from build123d import *

# Parameters (mm, degrees)
EXTRUDE_1_DEPTH = 2


with BuildPart() as part:
    # 草图2 → 凸台-拉伸1 (new body)
    with BuildSketch(Plane.XY):
        Polygon((-15.2, 6.5), (74.2, 6.5), (74.2, 8.5), (78, 8.5), (78, 6.5), (80.5, 6.5), (80.5, 4), (79, 4), (79, 1.4), (80.5, 1.4), (80.5, -1.6), (83.5, -1.6), (83.5, 1.4), (85, 1.4), (85, 4), (83.5, 4), (83.5, 6.5), (86, 6.5), (86, 8.5), (89.8, 8.5), (89.8, 6.5), (197.54, 6.5), (197.54, 8.5), (201.34, 8.5), (201.34, 6.5), (203.84, 6.5), (203.84, 4), (202.34, 4), (202.34, 1.4), (203.84, 1.4), (203.84, -1.6), (206.84, -1.6), (206.84, 1.4), (208.34, 1.4), (208.34, 4), (206.84, 4), (206.84, 6.5), (209.34, 6.5), (209.34, -27.5), (206.84, -27.5), (206.84, -25), (208.34, -25), (208.34, -22.4), (206.84, -22.4), (206.84, -19.4), (203.84, -19.4), (203.84, -22.4), (202.34, -22.4), (202.34, -25), (203.84, -25), (203.84, -27.5), (201.34, -27.5), (201.34, -29.5), (197.54, -29.5), (197.54, -27.5), (89.8, -27.5), (89.8, -29.5), (86, -29.5), (86, -27.5), (83.5, -27.5), (83.5, -25), (85, -25), (85, -22.4), (83.5, -22.4), (83.5, -19.4), (80.5, -19.4), (80.5, -22.4), (79, -22.4), (79, -25), (80.5, -25), (80.5, -27.5), (78, -27.5), (78, -29.5), (74.2, -29.5), (74.2, -27.5), (-15.2, -27.5), (-15.2, -29.5), (-19, -29.5), (-19, -27.5), (-21.5, -27.5), (-21.5, -25), (-20, -25), (-20, -22.4), (-21.5, -22.4), (-21.5, -19.4), (-24.5, -19.4), (-24.5, -22.4), (-26, -22.4), (-26, -25), (-24.5, -25), (-24.5, -27.5), (-27, -27.5), (-27, -29.5), (-30.8, -29.5), (-30.8, 8.5), (-27, 8.5), (-27, 6.5), (-24.5, 6.5), (-24.5, 4), (-26, 4), (-26, 1.4), (-24.5, 1.4), (-24.5, -1.6), (-21.5, -1.6), (-21.5, 1.4), (-20, 1.4), (-20, 4), (-21.5, 4), (-21.5, 6.5), (-19, 6.5), (-19, 8.5), (-15.2, 8.5), align=None)
        with BuildLine():
            Line((3.770961007, 2), (71.2, 2))
            ThreePointArc((71.2, 2), (71.907106781, 1.707106781), (72.2, 1))
            Line((72.2, 1), (72.2, -20.872954483))
            ThreePointArc((72.2, -20.872954483), (71.787980979, -21.681829238), (70.891443263, -21.824160423))
            Line((70.891443263, -21.824160423), (3.46240427, 0.04879406))
            ThreePointArc((3.46240427, 0.04879406), (2.783234845, 1.156195487), (3.770961007, 2))
        make_face(mode=Mode.SUBTRACT)
        with BuildLine():
            Line((92.8, 2), (174.852275232, 2))
            ThreePointArc((174.852275232, 2), (175.843645832, 1.131089029), (175.11219085, 0.034368667))
            Line((175.11219085, 0.034368667), (93.059915618, -22.051356057))
            ThreePointArc((93.059915618, -22.051356057), (92.191689067, -21.879423539), (91.8, -21.085724724))
            Line((91.8, -21.085724724), (91.8, 1))
            ThreePointArc((91.8, 1), (92.092893219, 1.707106781), (92.8, 2))
        make_face(mode=Mode.SUBTRACT)
        with BuildLine():
            Line((112.22780915, -21.034368667), (194.280084382, 1.051356057))
            ThreePointArc((194.280084382, 1.051356057), (195.148310933, 0.879423539), (195.54, 0.085724724))
            Line((195.54, 0.085724724), (195.54, -22))
            ThreePointArc((195.54, -22), (195.247106781, -22.707106781), (194.54, -23))
            Line((194.54, -23), (112.487724768, -23))
            ThreePointArc((112.487724768, -23), (111.496354168, -22.131089029), (112.22780915, -21.034368667))
        make_face(mode=Mode.SUBTRACT)
        with BuildLine():
            Line((-13.2, -0.127045517), (-13.2, -22))
            ThreePointArc((-13.2, -22), (-12.907106781, -22.707106781), (-12.2, -23))
            Line((-12.2, -23), (55.229038993, -23))
            ThreePointArc((55.229038993, -23), (56.216765155, -22.156195487), (55.53759573, -21.04879406))
            Line((55.53759573, -21.04879406), (-11.891443263, 0.824160423))
            ThreePointArc((-11.891443263, 0.824160423), (-12.787980979, 0.681829238), (-13.2, -0.127045517))
        make_face(mode=Mode.SUBTRACT)
    extrude(amount=EXTRUDE_1_DEPTH)


solid = part.part
Geometry: final body of the model. Coordinates: model frame, mm. A direction names the side the tool comes from. Round coordinates to 2 decimals unless told otherwise and drop trailing zeros. Loops run counter-clockwise (first coordinate to the right, second up) from the corner with the lowest first, then second, coordinate; pieces in that order, holes last.
Q1. Pull-direction query (Y, two-part tool) for faces 1 (the flat face through (91, -10, 2)), 2 (the flat face through (152.68, -10.146, 0.986)); classes: released by +Y, released by -Y, zero draft, split by the parting line, or undercut.
Q2. Pin query (flat end, axial travel): P1, Ø1, axis at x = 164, z = 1, coming from the -Y side; P2, Ø0.6, axis at y = 8, z = 1, coming from the +X side; P3, Ø1, axis at x = 207.5, z = 0.5, coming from the +Y side. Return the tip coordinate at first contact, or that it passes through.
Q3. Section B-B on x = 153. Return loops of the section in (y, z), plus the area to 3 significant figures.
Q4. Section A-A on y = -11. Return loops of the section in (x, z), plus the area to 3 significant figures.
Q5. Access query for faces 3 (the flat face through (91, -10, 0)), 4 (the flat face through (134.66, -10.854, 0.986)). Directions: +Z, -Z, +X, -X, +Y, -Y. A direction counts if a zero-diameter tool reaches every point of the face in a straight line with its end or side. Return the directions, or none.
Q6. Section C-C on z = 1.45. State how many separate pieces and enclosed holes the cut face has, plus the area to 3 significant figures.
Q7. Material intervals for L1, parallel to X at y = -26.5, z = 0.6; L2, parallel to Y at x = 71, z = 0.4; L3, parallel to Y at x = 29, z = 1.35, sorted ascending.
Evaluation:
1. face 1: zero draft
1. face 2: undercut
2. P1: stops at y = -27.5
2. P2: stops at x = 201.34
2. P3: stops at y = 6.5
3. outline: (-27.5, 0) - (-23, 0) - (-23, 2) - (-27.5, 2) - close; (-10.06, 0) - (-5.92, 0) - (-5.92, 2) - (-10.06, 2) - close; (2, 0) - (6.5, 0) - (6.5, 2) - (2, 2) - close
3. area: 26.3 mm2
4. outline: (-30.8, 0) - (-13.2, 0) - (-13.2, 2) - (-30.8, 2) - close; (24.56, 0) - (37.52, 0) - (37.52, 2) - (24.56, 2) - close; (72.2, 0) - (91.8, 0) - (91.8, 2) - (72.2, 2) - close; (134.12, 0) - (149.51, 0) - (149.51, 2) - (134.12, 2) - close; (195.54, 0) - (209.34, 0) - (209.34, 2) - (195.54, 2) - close
4. area: 159 mm2
5. face 3: -Z, +X, -X, +Y, -Y
5. face 4: +Z, -Z
6. separate pieces: 1
6. enclosed holes: 4
6. area: 4,050 mm2
7. L1: x = -30.8 to -24.5, -21.5 to 80.5, 83.5 to 203.84, 206.84 to 209.34
7. L2: y = -27.5 to -21.85, 2 to 6.5
7. L3: y = -27.5 to -23, -12.44 to -8.24, 2 to 6.5
